Here's how the part is built. I have some questions about the finished solid (model axes, mm). Face numbers are marked on the shaded views. A direction names the side the tool comes from. Coordinates: 2 decimals unless noted, no trailing zeros. Write each loop counter-clockwise with the first axis right and the second up, starting at its lowest first coordinate (ties: lowest second). Pieces come first, ordered by that corner, then holes. Notation, with made-up numbers: M 28.25,23.5 L 32.25,23.5 A16 ccw 32.25,50.5 Z; hole C 66,22.25 d9. An arc over 180 degrees is marked long. Use a Markdown table: item, result.
```python
from build123d import *

# Parameters (mm, degrees)
F0_R     = 6.6
F1_DEPTH = 9
F2_DEPTH = 7
F3_SIZE  = 2
F4_DEPTH = 3


with BuildPart() as f1:
    # F0 (on Top) → F1 (new body)
    with BuildSketch(Plane.XY):
        with BuildLine():
            ThreePointArc((1.338738724, 15.35871396), (-2.5323518967, 12.1283433891), (-7.5, 12.9903810568))
            ThreePointArc((-7.5, 12.9903810568), (-11.6205194267, 12.8362404515), (-12.6316670968, 8.838738724))
            ThreePointArc((-12.6316670968, 8.838738724), (-11.7696294292, 3.8710906207), (-15, 0))
            ThreePointArc((-15, 0), (-16.9267700334, -3.6455448029), (-13.9704058208, -6.519975236))
            ThreePointArc((-13.9704058208, -6.519975236), (-9.2372775325, -8.2572527684), (-7.5, -12.9903810568))
            ThreePointArc((-7.5, -12.9903810568), (-5.3062506067, -16.4817852544), (-1.338738724, -15.35871396))
            ThreePointArc((-1.338738724, -15.35871396), (2.5323518967, -12.1283433891), (7.5, -12.9903810568))
            ThreePointArc((7.5, -12.9903810568), (11.6205194267, -12.8362404515), (12.6316670968, -8.838738724))
            ThreePointArc((12.6316670968, -8.838738724), (11.7696294292, -3.8710906207), (15, 0))
            ThreePointArc((15, 0), (16.9267700334, 3.6455448029), (13.9704058208, 6.519975236))
            ThreePointArc((13.9704058208, 6.519975236), (9.2372775325, 8.2572527684), (7.5, 12.9903810568))
            ThreePointArc((7.5, 12.9903810568), (5.3062506067, 16.4817852544), (1.338738724, 15.35871396))
        make_face()
        Circle(F0_R, mode=Mode.SUBTRACT)
        Circle(F0_R)
        Polygon((-1.6743157806, -2.9), (-3.3486315613, 0), (-1.6743157806, 2.9), (1.6743157806, 2.9), (3.3486315613, 0), (1.6743157806, -2.9), align=None, mode=Mode.SUBTRACT)
        Polygon((-1.6743157806, 2.9), (-3.3486315613, 0), (-1.6743157806, -2.9), (1.6743157806, -2.9), (3.3486315613, 0), (1.6743157806, 2.9), align=None)
    extrude(amount=F1_DEPTH)

    # F0 (on Top) → F2 (cut)
    with BuildSketch(Plane.XY):
        Circle(F0_R)
        Polygon((-1.6743157806, -2.9), (-3.3486315613, 0), (-1.6743157806, 2.9), (1.6743157806, 2.9), (3.3486315613, 0), (1.6743157806, -2.9), align=None, mode=Mode.SUBTRACT)
    extrude(amount=F2_DEPTH, mode=Mode.SUBTRACT)

    # F3
    f3_edges = [f1.edges().sort_by_distance(p)[0] for p in [
        (-2.532352, 12.128343, 0),
        (5.306251, 16.481785, 0),
        (9.237278, 8.257253, 0),
        (16.92677, 3.645545, 0),
        (11.769629, -3.871091, 0),
        (2.532352, -12.128343, 0),
        (-5.306251, -16.481785, 0),
        (-9.237278, -8.257253, 0),
        (-16.92677, -3.645545, 0),
        (-11.769629, 3.871091, 0),
        (9.237278, 8.257253, 9),
        (5.306251, 16.481785, 9),
        (-2.532352, 12.128343, 9),
        (-11.620519, 12.83624, 9),
        (-11.769629, 3.871091, 9),
        (-16.92677, -3.645545, 9),
        (-9.237278, -8.257253, 9),
        (-5.306251, -16.481785, 9),
        (2.532352, -12.128343, 9),
        (11.620519, -12.83624, 9),
        (11.769629, -3.871091, 9),
        (16.92677, 3.645545, 9),
    ]]
    chamfer(f3_edges, length=F3_SIZE)

    # F0 (on Top) → F4 (cut)
    with BuildSketch(Plane.XY):
        Polygon((-1.6743157806, 2.9), (-3.3486315613, 0), (-1.6743157806, -2.9), (1.6743157806, -2.9), (3.3486315613, 0), (1.6743157806, 2.9), align=None)
    extrude(amount=F4_DEPTH, mode=Mode.SUBTRACT)


solid = f1.part
```
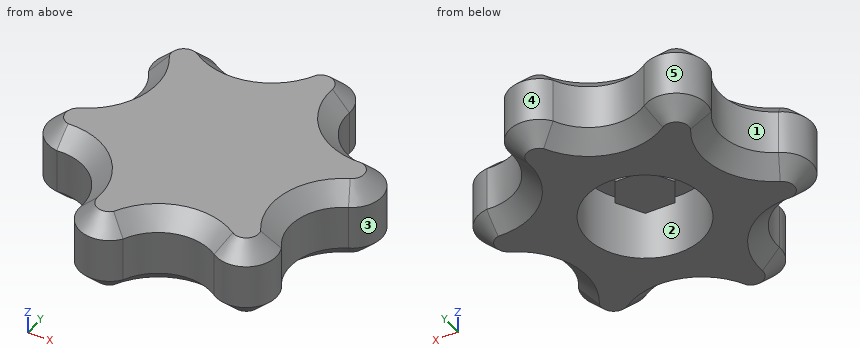
1. I need wall thicknesses on probe 1 along Y at (x, z) = (3, 4.5); probe 2 along Y at (x, z) = (0, 4.5); probe 3 along Z at (x, y) = (-3, -3). Which ranges of each line are inside material? Lowest first, please.
Answers follow:
| item | result |
|---|---|
| probe 1 | y = -12.02 to -5.88, -0.6 to 0.6, 5.88 to 16.54 |
| probe 2 | y = -13.53 to -6.6, -2.9 to 2.9, 6.6 to 13.53 |
| probe 3 | z = 7 to 9 |
2. We'd pull the mould along X, two halves only. Please class the marked faces 3, 4 and 5: +X half, -X half, draft (parallel to the pull), parting line (faces both ways), or undercut.
Answers follow:
| item | result |
|---|---|
| face 3 | +X half |
| face 4 | parting line |
| face 5 | undercut |
3. Which directions (+Z, -Z, +X, -X, +Y, -Y) give clear straight access to the entire face, cutting with the end or side of a thin tool? Please do the marked faces 1 and 2.
Answers follow:
| item | result |
|---|---|
| face 1 | +Z, -Z, -X |
| face 2 | -Z |
4. Will these pins go through, and if not, where does the flat tip stop? pin 1 Ø1.7 at (x, y) = (1, -0.5) entering from -Z; pin 2 Ø2 at (x, y) = (-4.5, -2.5) entering from -Z; pin 3 Ø1.5 at (y, z) = (1, 3) entering from +X.
Answers follow:
| item | result |
|---|---|
| pin 1 | stops at z = 3 |
| pin 2 | stops at z = 7 |
| pin 3 | stops at x = 16.69 |
5. Suppose I cut it at A-A on z = 6.5. Write out the boundary of the cut face in (x, y).
Answers follow:
| item | result |
|---|---|
| outline | M -15,0 A3.44 ccw -13.97,-6.52 A6 cw -7.5,-12.99 A3.44 ccw -1.34,-15.36 A6 cw 7.5,-12.99 A3.44 ccw 12.63,-8.84 A6 cw 15,0 A3.44 ccw 13.97,6.52 A6 cw 7.5,12.99 A3.44 ccw 1.34,15.36 A6 cw -7.5,12.99 A3.44 ccw -12.63,8.84 A6 cw Z; M -3.35,0 L -1.67,-2.9 L 1.67,-2.9 L 3.35,0 L 1.67,2.9 L -1.67,2.9 Z; hole C 0,0 d13.2 |
